Drawing for the job (mm, zero at the part's lowest x, y, z). Round coordinates to 2 decimals unless told otherwise and drop trailing zeros. Write each loop counter-clockwise with the first axis right and the second up, starting at its lowest first coordinate (ties: lowest second). Pieces come first, ordered by that corner, then holes.
Item 1: Band-saw the part on C-C, the plane z = 0.9. Write the cut outline in (x, y), then the cut area to 3 significant figures.
Item 2: Band-saw the part on A-A, the plane y = 75. Write the cut outline in (x, z), then the cut area to 3 significant figures.
Item 3: Band-saw the part on D-D, the plane y = 13. Write the cut outline in (x, z), then the cut area to 3 significant figures.
Item 4: Wall check: probe 1 along Y at (x, z) = (15, 1.3); probe 2 along X at (y, z) = (102.5, 1.9). Give the ranges that are in metal, low to high.
Item 5: Drop a flat-ended pin along its axis: pin 1 Ø4 at (x, y) = (15, 105) entering from +Z. Give the stop position or say it passes through.
Item 6: Band-saw the part on B-B, the plane x = 15. Write the cut outline in (y, z).
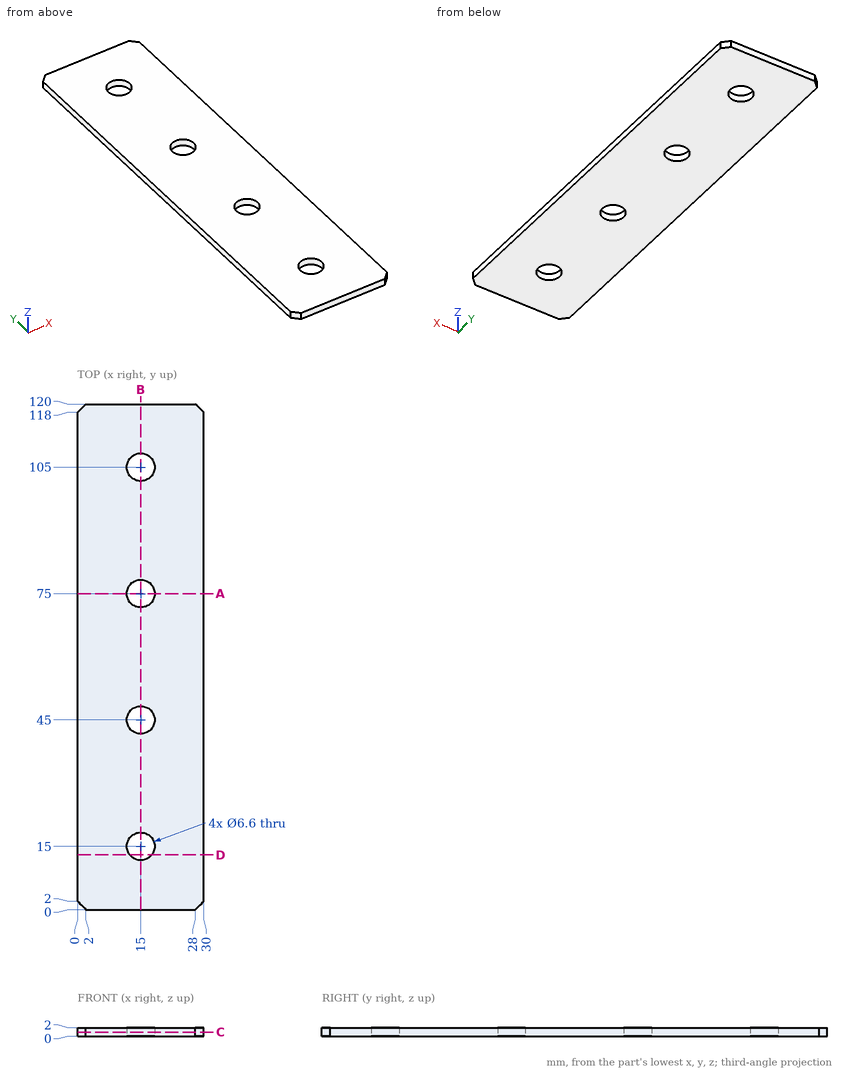
Results:
1. outline: (0, 2) - (2, 0) - (28, 0) - (30, 2) - (30, 118) - (28, 120) - (2, 120) - (0, 118) - close; hole circle Ø6.6 at (15, 15); hole circle Ø6.6 at (15, 45); hole circle Ø6.6 at (15, 75); hole circle Ø6.6 at (15, 105)
1. area: 3,460 mm2
2. outline: (0, 0) - (11.7, 0) - (11.7, 2) - (0, 2) - close; (18.3, 0) - (30, 0) - (30, 2) - (18.3, 2) - close
2. area: 46.8 mm2
3. outline: (0, 0) - (12.38, 0) - (12.38, 2) - (0, 2) - close; (17.62, 0) - (30, 0) - (30, 2) - (17.62, 2) - close
3. area: 49.5 mm2
4. probe 1: y = 0 to 11.7, 18.3 to 41.7, 48.3 to 71.7, 78.3 to 101.7, 108.3 to 120
4. probe 2: x = 0 to 12.85, 17.15 to 30
5. pin 1: passes through
6. outline: (0, 0) - (11.7, 0) - (11.7, 2) - (0, 2) - close; (18.3, 0) - (41.7, 0) - (41.7, 2) - (18.3, 2) - close; (48.3, 0) - (71.7, 0) - (71.7, 2) - (48.3, 2) - close; (78.3, 0) - (101.7, 0) - (101.7, 2) - (78.3, 2) - close; (108.3, 0) - (120, 0) - (120, 2) - (108.3, 2) - close
